Autodesk Fusion 360 part; units mm, degrees
sketch "Sketch1" plane through (0, 0, 0) normal (0, 0, 1) x (1, 0, 0)
  line L0 (61.42, -42.3) -> (-56.55, -42.3)
  line L1 (-63.55, -35.3) -> (-63.55, 35.3)
  line L2 (-56.55, 42.3) -> (61.42, 42.3)
  line L3 (63.55, 40.17) -> (63.55, -40.17)
  line L4 (63.55, -42.3) -> (-63.55, 42.3) construction
  line L5 (-63.55, -42.3) -> (63.55, 42.3) construction
  line L6 (-56.55, 42.3) -> (-63.55, 35.3)
  line L7 (0, -42.3) -> (0, 42.3) construction
  line L8 (63.55, 0) -> (-63.55, 0) construction
  line L9 (-56.55, -42.3) -> (-63.55, -35.3)
  arc A0 (63.55, 40.17) -> (61.42, 42.3) centre (61.42, 40.17) ccw
  arc A1 (61.42, -42.3) -> (63.55, -40.17) centre (61.42, -40.17) ccw
  dimension "d1" = 84.6
  dimension "d2" = 127.1
  dimension "d3" = 7
  dimension "d4" = 7
  dimension "d5" = 2.13
extrude "Extrude1" add sketch "Sketch1" against normal blind 9
sketch "Sketch2" plane through (0, 0, -9) normal (0, 0, -1) x (1, 0, 0)
  line L0 (61.42, 42.3) -> (-56.55, 42.3)
  line L1 (-56.55, 42.3) -> (-63.55, 35.3)
  line L2 (-63.55, 35.3) -> (-63.55, -35.3)
  line L3 (-63.55, -35.3) -> (-56.55, -42.3)
  line L4 (-56.55, -42.3) -> (61.42, -42.3)
  arc A0 (61.42, -42.3) -> (63.55, -40.17) centre (61.42, -40.17) ccw
  line L5 (63.55, -40.17) -> (63.55, 40.17)
  arc A1 (63.55, 40.17) -> (61.42, 42.3) centre (61.42, 40.17) ccw
  line L6 (61.42, -41.3) -> (-56.1358, -41.3)
  line L7 (-62.55, -34.8858) -> (-62.55, 34.8858)
  line L8 (-56.1358, 41.3) -> (61.42, 41.3)
  line L9 (62.55, 40.17) -> (62.55, -40.17)
  line L10 (62.55, -41.3) -> (-62.55, 41.3) construction
  line L11 (-62.55, -41.3) -> (62.55, 41.3) construction
  line L12 (-56.1358, 41.3) -> (-62.55, 34.8858)
  arc A2 (62.55, 40.17) -> (61.42, 41.3) centre (61.42, 40.17) ccw
  line L13 (63.55, 0) -> (-63.55, 0) construction
  line L14 (-56.1358, -41.3) -> (-62.55, -34.8858)
  arc A3 (61.42, -41.3) -> (62.55, -40.17) centre (61.42, -40.17) ccw
  dimension "d8" = 125.1
  dimension "d9" = 82.6
  dimension "d10" = 6.4142
  dimension "d11" = 6.4142
  dimension "d12" = 1
  dimension "d13" = 1.13
extrude "Extrude2" cut sketch "Sketch2" against normal blind 8 contours L6 L7 L8 L9 L12 A2 L14 A3
sketch "Sketch3" plane through (0, 0, -1) normal (0, 0, -1) x (1, 0, 0)
  line L0 (-56.1358, -41.3) -> (61.42, -41.3)
  arc A0 (61.42, -41.3) -> (62.55, -40.17) centre (61.42, -40.17) ccw
  line L1 (62.55, -40.17) -> (62.55, 40.17)
  arc A1 (62.55, 40.17) -> (61.42, 41.3) centre (61.42, 40.17) ccw
  line L2 (61.42, 41.3) -> (-56.1358, 41.3)
  line L3 (-56.1358, 41.3) -> (-62.55, 34.8858)
  line L4 (-62.55, 34.8858) -> (-62.55, -34.8858)
  line L5 (-62.55, -34.8858) -> (-56.1358, -41.3)
  line L6 (-62.55, 32.8642) -> (-35.55, 32.8642) construction
  line L7 (-35.55, 32.8642) -> (-35.55, 41.3) construction
  line L8 (-35.55, 41.3) -> (-36.55, 41.3)
  line L9 (-36.55, 41.3) -> (-36.55, 37.5)
  line L10 (-36.55, 37.5) -> (-35.55, 37.5)
  line L11 (-35.55, 37.5) -> (-35.55, 41.3)
  line L12 (-50.2731, 41.3) -> (-50.2731, 26.6) construction
  line L13 (-50.2731, 26.6) -> (-62.55, 26.6) construction
  line L14 (-62.55, 26.6) -> (-58.75, 26.6)
  line L15 (-58.75, 26.6) -> (-58.75, 27.6)
  line L16 (-58.75, 27.6) -> (-62.55, 27.6)
  line L17 (-62.55, 27.6) -> (-62.55, 26.6)
  line L18 (62.55, 0) -> (-62.55, 0) construction
  line L19 (-62.55, 30.673) -> (-62.55, 55) construction
  line L20 (62.55, 34.8173) -> (62.55, 55) construction
  line L21 (62.55, 55) -> (-62.55, 55) construction
  line L22 (0, 55) -> (0, -41.3) construction
  line L23 (62.55, 27.6) -> (62.55, 26.6)
  line L24 (62.55, 26.6) -> (58.75, 26.6)
  line L25 (58.75, 27.6) -> (62.55, 27.6)
  line L26 (58.75, 26.6) -> (58.75, 27.6)
  line L27 (36.55, 41.3) -> (36.55, 37.5)
  line L28 (35.55, 37.5) -> (35.55, 41.3)
  line L29 (36.55, 37.5) -> (35.55, 37.5)
  line L30 (35.55, 41.3) -> (36.55, 41.3)
  line L31 (62.55, -26.6) -> (58.75, -26.6)
  line L32 (58.75, -27.6) -> (62.55, -27.6)
  line L33 (58.75, -26.6) -> (58.75, -27.6)
  line L34 (35.55, -37.5) -> (35.55, -41.3)
  line L35 (36.55, -37.5) -> (35.55, -37.5)
  line L36 (36.55, -41.3) -> (36.55, -37.5)
  line L37 (62.55, -27.6) -> (62.55, -26.6)
  line L38 (35.55, -41.3) -> (36.55, -41.3)
  line L39 (-58.75, -26.6) -> (-58.75, -27.6)
  line L40 (-62.55, -26.6) -> (-58.75, -26.6)
  line L41 (-58.75, -27.6) -> (-62.55, -27.6)
  line L42 (-62.55, -27.6) -> (-62.55, -26.6)
  line L43 (-36.55, -37.5) -> (-35.55, -37.5)
  line L44 (-35.55, -37.5) -> (-35.55, -41.3)
  line L45 (-36.55, -41.3) -> (-36.55, -37.5)
  line L46 (-35.55, -41.3) -> (-36.55, -41.3)
  dimension "d16" = 27
  dimension "d17" = 3.8
  dimension "d18" = 1
  dimension "d19" = 14.7
  dimension "d20" = 3.8
  dimension "d21" = 1
extrude "Extrude3" add sketch "Sketch3" along normal blind 1 contours L0 L43 L44 L45 L46 | L4 L39 L40 L41 L42 | L0 L34 L35 L36 L38 | L4 L14 L15 L16 L17 | L1 L31 L32 L33 L37 | L2 L8 L9 L10 L11 | L1 L23 L24 L25 L26 | L2 L27 L28 L29 L30
sketch "Sketch4" plane through (0, 0, 0) normal (0, 0, 1) x (-1, 0, 0)
  line L0 (56.55, 42.3) -> (-61.42, 42.3)
  arc A0 (-61.42, 42.3) -> (-63.55, 40.17) centre (-61.42, 40.17) ccw
  line L1 (-63.55, 40.17) -> (-63.55, -40.17)
  arc A1 (-63.55, -40.17) -> (-61.42, -42.3) centre (-61.42, -40.17) ccw
  line L2 (-61.42, -42.3) -> (56.55, -42.3)
  line L3 (56.55, -42.3) -> (63.55, -35.3)
  line L4 (63.55, -35.3) -> (63.55, 35.3)
  line L5 (63.55, 35.3) -> (56.55, 42.3)
  line L6 (-63.55, -34.3916) -> (-62.25, -34.3916) construction
  line L7 (-62.25, -34.3916) -> (-62.25, -36.4) construction
  line L8 (-60, -42.3) -> (-66.2, -42.3) construction
  line L9 (-63.55, -39.2433) -> (-63.55, -43.1) construction
  line L10 (-62.25, -36.4) -> (-60.95, -36.4)
  line L11 (-60.95, -36.4) -> (-60.95, 36.4)
  line L12 (-60.95, 36.4) -> (-62.25, 36.4)
  line L13 (-62.25, 36.4) -> (-62.25, -36.4)
  line L14 (-52.6219, -42.3) -> (-52.6219, -41) construction
  line L15 (-52.6219, -41) -> (-57.65, -41) construction
  line L16 (-57.65, -41) -> (53.05, -41)
  line L17 (53.05, -41) -> (53.05, -39.7)
  line L18 (53.05, -39.7) -> (-57.65, -39.7)
  line L19 (-57.65, -39.7) -> (-57.65, -41)
  line L20 (53.05, 39.7) -> (-57.65, 39.7)
  line L21 (-57.65, 41) -> (53.05, 41)
  line L22 (-57.65, 39.7) -> (-57.65, 41)
  line L23 (53.05, 41) -> (53.05, 39.7)
  line L24 (60.95, 0) -> (60.95, -32.3)
  line L25 (60.95, -32.3) -> (62.25, -32.3)
  line L26 (62.25, -32.3) -> (62.25, 0)
  line L27 (60.95, 0) -> (60.95, 32.3)
  line L28 (62.25, 32.3) -> (62.25, 0)
  line L29 (60.95, 32.3) -> (62.25, 32.3)
  line L30 (-63.55, 0) -> (60.95, 0) construction
  line L31 (62.25, 0) -> (63.55, 0) construction
  dimension "d24" = 1.3
  dimension "d25" = 5.9
  dimension "d26" = 72.8
  dimension "d27" = 1.3
  dimension "d28" = 1.3
  dimension "d29" = 5.9
  dimension "d30" = 1.3
  dimension "d31" = 110.7
  dimension "d32" = 32.3
  dimension "d33" = 1.3
  dimension "d34" = 1.3
extrude "Extrude4" add sketch "Sketch4" along normal blind 1 contours L10 L11 L12 L13 | L16 L17 L18 L19 | L20 L21 L22 L23 | L24 L25 L26 L27 L28 L29
equation "d4 = d3"
equation "d11 = d10"
Here's how the part is built. I have some questions about the finished solid (model axes, mm). A direction names the side the tool comes from. Coordinates: 2 decimals unless noted, no trailing zeros. Order: outer loops, then holes, each group sorted by start corner. A loop starts at its lowest first (then second) coordinate and runs counter-clockwise, first axis right, second up. Notation, with made-up numbers: M 7,87 L 34,87 A9 cw 34,103 Z; hole C -18.75,62 d5. An arc over 180 degrees is marked long. Answer as CSV lines item,"result". Start each with the question number.
1. I want a section at C-C, the plane x = -7. Write out the boundary of the cut face in (y, z).
2. I want a section at A-A, the plane y = -29. Write out the boundary of the cut face in (x, z), and give its area (3 significant figures).
3. I want a section at B-B, the plane z = -7.5. Write out the boundary of the cut face in (x, y).
4. For pin 1 (25 mm diameter, centred on x = -19.5, y = -17, fed in from -Z); pin 2 (3 mm diameter, centred on x = -50.5, y = -11, fed in from +Z); pin 3 (0.5 mm diameter, centred on y = -40, z = 0.5, fed in from -X), each with a flat end and sliding along its axis, tell me the tip position at first contact or that it passes through.
5. We'd pull the mould along X, two halves only. Please class faces 3 (the flat face through (3, 41.3, -5)), 4 (the flat face through (63.55, 1, -4)), 5 (the flat face through (3, -42.3, -4)): released by +X, released by -X, zero draft, split by the parting line, or undercut.
6. On a 3-axis mill with a long thin cutter (end or side, diameter ignored), from which of +Z, -Z, +X, -X, +Y, -Y can I reach the whole of each face in a straight line? I mean faces 1 (the flat face through (-63.55, 0, -4)), 2 (the flat face through (-59.298, -38.138, -5.056)). Say none if no direction works.
7. I need wall thicknesses on line 1 (X direction, y = 1, z = -7.5); line 2 (Y direction, x = 28.5, z = -2.5); line 3 (X direction, y = 38, z = -1.5). Which ranges of each line are inside material? Lowest first, please. Write a range as [from, to].
Recorded:
1,outline,"M -42.3,-9 L -41.3,-9 L -41.3,-1 L 41.3,-1 L 41.3,-9 L 42.3,-9 L 42.3,0 L 41,0 L 41,1 L 39.7,1 L 39.7,0 L -39.7,0 L -39.7,1 L -41,1 L -41,0 L -42.3,0 Z"
2,outline,"M -63.55,-9 L -62.55,-9 L -62.55,-1 L 62.55,-1 L 62.55,-9 L 63.55,-9 L 63.55,0 L 62.25,0 L 62.25,1 L 60.95,1 L 60.95,0 L -60.95,0 L -60.95,1 L -62.25,1 L -62.25,0 L -63.55,0 Z"
2,area,"146 mm2"
3,outline,"M -63.55,-35.3 L -56.55,-42.3 L 61.42,-42.3 A2.13 ccw 63.55,-40.17 L 63.55,40.17 A2.13 ccw 61.42,42.3 L -56.55,42.3 L -63.55,35.3 Z; hole M -62.55,-34.89 L -56.14,-41.3 L 61.42,-41.3 A1.13 ccw 62.55,-40.17 L 62.55,40.17 A1.13 ccw 61.42,41.3 L -56.14,41.3 L -62.55,34.89 Z"
4,pin 1,"stops at z = -1"
4,pin 2,"stops at z = 0"
4,pin 3,"stops at x = -53.05"
5,face 3,"undercut"
5,face 4,"released by +X"
5,face 5,"zero draft"
6,face 1,"+Z, -Z, -X, +Y, -Y"
6,face 2,"-Z"
7,line 1,"x = [-63.55, -62.55], [62.55, 63.55]"
7,line 2,"y = [-42.3, -41.3], [41.3, 42.3]"
7,line 3,"x = [-60.85, -59.44], [-36.55, -35.55], [35.55, 36.55], [62.55, 63.55]"
